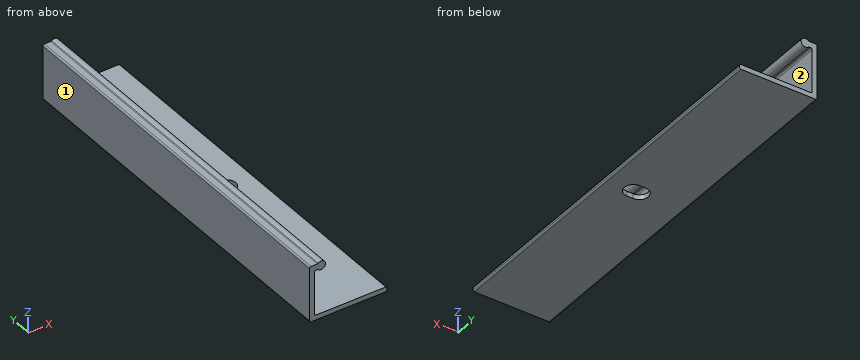
```python
from build123d import *

# Parameters (mm, degrees)
BOSS_EXTRUDE1_DEPTH = 50.8
CUT_EXTRUDE1_DEPTH  = 2.27


with BuildPart() as part:
    # Sketch2 → Boss-Extrude1 (new body, symmetric)
    with BuildSketch(Plane(origin=(0, 0, 0), x_dir=(1, 0, 0), z_dir=(0, 1, 0))):
        with BuildLine():
            Line((0.381, 0), (20.066, 0))
            ThreePointArc((20.066, 0), (20.335407684, -0.111592316), (20.447, -0.381))
            Line((20.447, -0.381), (20.447, -0.889))
            ThreePointArc((20.447, -0.889), (20.335407684, -1.158407684), (20.066, -1.27))
            Line((20.066, -1.27), (1.651, -1.27))
            ThreePointArc((1.651, -1.27), (1.381592316, -1.381592316), (1.27, -1.651))
            Line((1.27, -1.651), (1.27, -12.827))
            ThreePointArc((1.27, -12.827), (1.381592316, -13.096407684), (1.651, -13.208))
            Line((1.651, -13.208), (2.03996875, -13.208))
            ThreePointArc((2.03996875, -13.208), (2.174672592, -13.183392866), (2.291976563, -13.11275))
            ThreePointArc((2.291976563, -13.11275), (4.191, -13.97), (2.291976563, -14.82725))
            ThreePointArc((2.291976563, -14.82725), (2.174672592, -14.756607134), (2.03996875, -14.732))
            Line((2.03996875, -14.732), (0.381, -14.732))
            ThreePointArc((0.381, -14.732), (0.111592316, -14.620407684), (0, -14.351))
            Line((0, -14.351), (0, -0.381))
            ThreePointArc((0, -0.381), (0.111592316, -0.111592316), (0.381, 0))
        make_face()
    extrude(amount=BOSS_EXTRUDE1_DEPTH, both=True)

    # Sketch7 → Cut-Extrude1 (cut, through all)
    with BuildSketch(Plane.XY.offset(1.27)):
        with BuildLine():
            Line((11.71575, 2.38125), (13.30325, 2.38125))
            ThreePointArc((13.30325, 2.38125), (15.6845, 0), (13.30325, -2.38125))
            Line((13.30325, -2.38125), (11.71575, -2.38125))
            ThreePointArc((11.71575, -2.38125), (9.3345, 0), (11.71575, 2.38125))
        make_face()
    extrude(amount=-CUT_EXTRUDE1_DEPTH, mode=Mode.SUBTRACT)


solid = part.part
```
Model file for the job. Use its own axes, mm. Face numbers are marked on the shaded views. A direction names the side the tool comes from. Coordinates: 2 decimals unless noted, no trailing zeros. Loops run counter-clockwise (first coordinate to the right, second up) from the corner with the lowest first, then second, coordinate; pieces in that order, holes last. Notation, with made-up numbers: (86.25, -0.75) - (131.25, -0.75) arc R24 cw to (131.25, 38.25) - close; hole circle Ø6 at (57.5, 24.25). An arc over 180 degrees is marked (long way). Answer as a JSON object with one key per item and string values. Group by question number.
(1) Flat gauge pins, fed straight in: pin 1 (5 mm diameter, centred on x = 16, y = -18.5, fed in from +Z); pin 2 (3.5 mm diameter, centred on y = -3.5, z = 7.5, fed in from +X); pin 3 (3 mm diameter, centred on y = 1, z = 13, fed in from +X). Where does each tip first touch, or does it go through?
(2) Probe line 1 along Z through (x, y) = (1.75, 0.5); line 2 along Z through (x, y) = (16.25, 22.5). List the from-to ranges inside material, lowest first.
(3) Tool access for the marked faces 1 and 2: list every direction of +Z, -Z, +X, -X, +Y, -Y with a clear straight run to the whole face (end or side of a thin tool).
(4) Cut at A-A (y = 0). Give the cut face in (x, z), then the cut area to 3 significant figures.
(5) Cut at D-D (z = 3). Give the cut face in (x, y).
(6) Cut at C-C (y = -37). Give the cut face in (x, z), then the cut area to 3 significant figures.
(7) Cut at B-B (x = 14.25). Give the cut face in (y, z).
Geometry says:
{
 "1": {"pin 1": "stops at z = 1.27", "pin 2": "stops at x = 1.27", "pin 3": "stops at x = 4.19"},
 "2": {"line 1": "z = 0 to 1.27, 13.21 to 14.73", "line 2": "z = 0 to 1.27"},
 "3": {"face 1": "+Z, -Z, -X, +Y, -Y", "face 2": "+X, +Y, -Y"},
 "4": {"outline": "(0, 0.38) arc R0.38 ccw to (0.38, 0) - (9.33, 0) - (9.33, 1.27) - (1.65, 1.27) arc R0.38 cw to (1.27, 1.65) - (1.27, 12.83) arc R0.38 cw to (1.65, 13.21) - (2.04, 13.21) arc R0.38 cw to (2.29, 13.11) arc R1.14 ccw (long way) to (2.29, 14.83) arc R0.38 cw to (2.04, 14.73) - (0.38, 14.73) arc R0.38 ccw to (0, 14.35) - close; (15.68, 0) - (20.07, 0) arc R0.38 ccw to (20.45, 0.38) - (20.45, 0.89) arc R0.38 ccw to (20.07, 1.27) - (15.68, 1.27) - close", "area": "40.2 mm^2"},
 "5": {"outline": "(0, -50.8) - (1.27, -50.8) - (1.27, 50.8) - (0, 50.8) - close"},
 "6": {"outline": "(0, 0.38) arc R0.38 ccw to (0.38, 0) - (20.07, 0) arc R0.38 ccw to (20.45, 0.38) - (20.45, 0.89) arc R0.38 ccw to (20.07, 1.27) - (1.65, 1.27) arc R0.38 cw to (1.27, 1.65) - (1.27, 12.83) arc R0.38 cw to (1.65, 13.21) - (2.04, 13.21) arc R0.38 cw to (2.29, 13.11) arc R1.14 ccw (long way) to (2.29, 14.83) arc R0.38 cw to (2.04, 14.73) - (0.38, 14.73) arc R0.38 ccw to (0, 14.35) - close", "area": "48.2 mm^2"},
 "7": {"outline": "(-50.8, 0) - (-2.18, 0) - (-2.18, 1.27) - (-50.8, 1.27) - close; (2.18, 0) - (50.8, 0) - (50.8, 1.27) - (2.18, 1.27) - close"}
}
